Build history of the part. All positions in model axes, mm. A direction names the side the tool comes from. Give positions to 0.01 mm unless a question says otherwise; leave off trailing zeros. Write each loop counter-clockwise with the first axis right and the second up, starting at its lowest first coordinate (ties: lowest second). Pieces come first, ordered by that corner, then holes. Notation, with made-up numbers: M 40,26 L 79,26 A20 cw 79,63 Z; hole C 76,79.25 d6. An arc over 180 degrees is marked long. Return JSON: item names as keys, results as strings. Group by question number.
Q1. Flat gauge pins, fed straight in: pin 1 Ø5 at (y, z) = (-24.5, -1) entering from +X; pin 2 Ø1.4 at (x, y) = (1.5, -19.5) entering from +Z; pin 3 Ø1.5 at (x, z) = (2, 7.5) entering from -Y; pin 4 Ø1.4 at (y, z) = (-12.5, -2) entering from -X. Where does each tip first touch, or does it go through?
Q2. Band-saw the part on B-B, the plane x = 8. Give the cut face in (y, z), then the cut area to 3 significant figures.
Q3. Band-saw the part on A-A, the plane z = -7.75. Give the cut face in (x, y), then the cut area to 3 significant figures.
Q4. Pull direction X, two halves, no side cores. Call faces 4 (the flat face through (-10, -20, -6)), 5 (the cylindrical face through (9.699, -19.72, -9.715)), 6 (the flat face through (2, -20, -4.7)): +X half, -X half, draft (parallel to the pull), parting line (faces both ways), or undercut.
Q5. Tool access for faces 1 (the flat face through (-9, -20, 3)), 2 (the flat face through (-6, -20, 8)), 3 (the flat face through (3, -20, 9)): list every direction of +Z, -Z, +X, -X, +Y, -Y with a clear straight run to the whole face (end or side of a thin tool).
Q6. Wall check: probe 1 along Z at (x, y) = (-8.75, -10); probe 2 along X at (y, z) = (-32.5, 3.75); probe 3 along Z at (x, y) = (-5.75, -38). Give the ranges that are in metal, low to high.
from build123d import *

# Parameters (mm, degrees)
PAD_DEPTH          = 40
POCKET_DEPTH       = 380
POLARPATTERN_COUNT = 4
POCKET001_DEPTH    = 380


with BuildPart() as part:
    # Sketch → Pad (new body)
    with BuildSketch(Plane.XZ):
        with BuildLine():
            Line((-9, 10), (9, 10))
            ThreePointArc((10, 9), (9.707107, 9.707107), (9, 10))
            Line((10, 9), (10, -9))
            ThreePointArc((9, -10), (9.707107, -9.707107), (10, -9))
            Line((9, -10), (-9, -10))
            ThreePointArc((-10, -9), (-9.707107, -9.707107), (-9, -10))
            Line((-10, -9), (-10, 9))
            ThreePointArc((-9, 10), (-9.707107, 9.707107), (-10, 9))
        make_face()
    extrude(amount=PAD_DEPTH)

    # Sketch001 (on Face10 of Pad) → Pocket (cut)
    with BuildSketch(Plane.XZ.offset(40)):
        Polygon((-3.4, 10), (-3.4, 9.6), (-3, 9.6), (-3, 8.5), (-6, 8.5), (-6, 7), (-3.35, 4.7), (-0.65, 4.7), (0, 4.3), (0.65, 4.7), (3.35, 4.7), (6, 7), (6, 8.5), (3, 8.5), (3, 9.6), (3.4, 9.6), (3.4, 10), align=None)
    pocket = extrude(amount=-POCKET_DEPTH, mode=Mode.SUBTRACT)

    # PolarPattern: Pocket ×4 about axis
    polarpattern_axis = Axis((0, -40, 0), (0, -1, 0))
    for i in range(1, POLARPATTERN_COUNT):
        add(pocket.rotate(polarpattern_axis, i * 360 / POLARPATTERN_COUNT), mode=Mode.SUBTRACT)

    # Sketch002 (on Face4 of PolarPattern) → Pocket001 (cut)
    with BuildSketch(Plane.XZ.offset(40)):
        with BuildLine():
            ThreePointArc((1.340499, 2.401159), (0, 2.75), (-1.340499, 2.401159))
            Line((-1.944544, 3.005204), (-1.340499, 2.401159))
            Line((-3.005204, 1.944544), (-1.944544, 3.005204))
            Line((-2.401159, 1.340499), (-3.005204, 1.944544))
            ThreePointArc((-2.401159, 1.340499), (-2.75, 0), (-2.401159, -1.340499))
            Line((-3.005204, -1.944544), (-2.401159, -1.340499))
            Line((-1.944544, -3.005204), (-3.005204, -1.944544))
            Line((-1.340499, -2.401159), (-1.944544, -3.005204))
            ThreePointArc((-1.340499, -2.401159), (0, -2.75), (1.340499, -2.401159))
            Line((1.944544, -3.005204), (1.340499, -2.401159))
            Line((3.005204, -1.944544), (1.944544, -3.005204))
            Line((2.401159, -1.340499), (3.005204, -1.944544))
            ThreePointArc((2.401159, -1.340499), (2.75, 0), (2.401159, 1.340499))
            Line((2.401159, 1.340499), (3.005204, 1.944544))
            Line((3.005204, 1.944544), (1.944544, 3.005204))
            Line((1.944544, 3.005204), (1.340499, 2.401159))
        make_face()
    extrude(amount=-POCKET001_DEPTH, mode=Mode.SUBTRACT)


solid = part.part
From the geometry:
{
 "1": {"pin 1": "stops at x = 10", "pin 2": "stops at z = 4.7", "pin 3": "passes through", "pin 4": "stops at x = -4.7"},
 "2": {"outline": "M -40,-10 L 0,-10 L 0,-6 L -40,-6 Z; M -40,6 L 0,6 L 0,10 L -40,10 Z", "area": "320 mm^2"},
 "3": {"outline": "M -10,-40 L -6,-40 L -6,0 L -10,0 Z; M 6,-40 L 10,-40 L 10,0 L 6,0 Z", "area": "320 mm^2"},
 "4": {"face 4": "-X half", "face 5": "+X half", "face 6": "undercut"},
 "5": {"face 1": "-X, +Y, -Y", "face 2": "+Y, -Y", "face 3": "+Z, +Y, -Y"},
 "6": {"probe 1": "z = -10 to -3, 3 to 10", "probe 2": "x = -10 to -8.5, -5.05 to 5.05, 8.5 to 10", "probe 3": "z = -10 to -8.5, -6.78 to -4.56, 4.56 to 6.78, 8.5 to 10"}
}
